The listing builds one solid part. Answer for the finished solid, in the listing's coordinates (mm). A direction names the side the tool comes from. Coordinates: 2 decimals unless noted, no trailing zeros. Order: outer loops, then holes, each group sorted by start corner. A loop starts at its lowest first (then second) coordinate and runs counter-clockwise, first axis right, second up.
```python
from build123d import *

# Parameters (mm, degrees)
FLANGE_HOLES_D    = 2.8702
DOWEL_HOLES_D     = 4.7625
DOWEL_HOLES_DEPTH = 6.35
DOWEL_HOLES_TIP   = 1.430799349
FILLET1_R         = 8.89
CHAMFER1_SIZE     = 2.141545552
CHAMFER1_SIZE_2   = 2.54


with BuildPart() as part:
    # Sketch2 → Main Structure (revolve)
    with BuildSketch(Plane.XY, mode=Mode.PRIVATE) as main_structure_sk:
        Polygon((0, 20.583496156), (0, 56.35625), (9.525, 56.35625), (9.525, 16.256), (66.806461084, 16.256), (139.7, 31.75), (139.7, 29.592458901), (60.325, 12.720781818), (60.325, 14.351), (10.795, 14.351), align=None)
    revolve(main_structure_sk.sketch.rotate(Axis((0, 0, 0), (1, 0, 0)), 90), axis=Axis((0, 0, 0), (1, 0, 0)))

    # Flange Holes (through all)
    with Locations(Plane.ZY):
        with Locations((0, -51.6255), (-25.81275, -44.708994483), (-44.708994483, -25.81275), (-51.6255, 0), (-44.708994483, 25.81275), (-25.81275, 44.708994483), (0, 51.6255), (25.81275, 44.708994483), (44.708994483, 25.81275), (51.6255, 0), (44.708994483, -25.81275), (25.81275, -44.708994483)):
            Hole(FLANGE_HOLES_D / 2)

    # Dowel Holes
    with Locations(Plane.ZY):
        with Locations((49.866403745, -13.361662613), (-49.866403745, 13.361662613)):
            Hole(DOWEL_HOLES_D / 2, depth=DOWEL_HOLES_DEPTH)
            with Locations((0, 0, -(DOWEL_HOLES_DEPTH + DOWEL_HOLES_TIP / 2))):  # 118° drill point
                Cone(0, DOWEL_HOLES_D / 2, DOWEL_HOLES_TIP, mode=Mode.SUBTRACT)

    # Fillet1
    fillet1_edges = [part.edges().sort_by_distance(p)[0] for p in [
        (66.806461084, 0, -16.256),
        (9.525, 0, -16.256),
    ]]
    fillet(fillet1_edges, radius=FILLET1_R)

    # Sketch13 → Cut-Revolve1 (revolve, cut)
    with BuildSketch(Plane(origin=(0, 0, 0), x_dir=(1, 0, 0), z_dir=(0, 1, 0)), mode=Mode.PRIVATE) as cut_revolve1_sk:
        Polygon((0, 38.1), (3.33331808, 0), (0, 0), align=None)
    revolve(cut_revolve1_sk.sketch.rotate(Axis((3.33331808, 0, 0), (-1, 0, 0)), 180), axis=Axis((3.33331808, 0, 0), (-1, 0, 0)), mode=Mode.SUBTRACT)

    # Chamfer1
    # the kernel refuses this chamfer: 3.297690964, 2.54, 2.141545552 mm, written as the material it takes off along each edge
    with BuildSketch(Plane(origin=(139.7, 0, 0), x_dir=(0, 0, 1), z_dir=(0, 1, 0))) as chamfer1_piece_1:
        Polygon((31.75 - CHAMFER1_SIZE * 0.207911690799, -CHAMFER1_SIZE * 0.978147600645), (31.75 - CHAMFER1_SIZE_2, 0), (31.75, 0), align=None)
    revolve(axis=Axis((139.7, 0, 0), (1, 0, 0)), mode=Mode.SUBTRACT)


solid = part.part
```
(1) Find section B-B (x = 16.5). Write down the section's boundary in (y, z), and give its area (3 significant figures).
(2) Each of these flat-tipped pins is pushed along its axis until it touches: pin 1 Ø10 at (y, z) = (-4, 13.5) entering from -X; pin 2 Ø23 at (y, z) = (4, -5.5) entering from -X; pin 3 Ø2.5 at (y, z) = (25.81, 44.71) entering from +X; pin 4 Ø4.5 at (y, z) = (25.81, -44.71) entering from +X (3 decimals). Where does it stop, or does it pass through?
(3) Find section A-A (x = 85). Write down the section's boundary in (y, z).
(4) The mould has two halves that part along Y. Classify faces 1 (the face through (9.525, 12, 24)), 2 (the face through (4.829, 34.292, -44.722)), 3 (the face through (60.325, 13, 1)): released by +Y, released by -Y, zero draft, split by the parting line, or undercut.
(5) Consider line 1 (X direction, y = -33, z = 18.5) (3 decimals); line 2 (Y direction, x = 68.5, z = 10); line 3 (Z direction, x = 43.5, y = 6). Determine where each line is inside the solid, lowest interval first.
(6) For faces 4 (the face through (99.3, 12.78, -16.67)), 5 (the face through (3.22, -11.35, 48.59)), 6 (the face through (95.387, 19.811, 10.304)), determine the directions among +Z, -Z, +X, -X, +Y, -Y from which every point of the face is accessible in a straight line to the end or side of a thin tool.
Findings below:
1. outline: circle Ø32.93 at (0, 0); hole circle Ø28.7 at (0, 0)
1. area: 205 mm2
2. pin 1: stops at x = 2.6
2. pin 2: stops at x = 3.95
2. pin 3: passes through
2. pin 4: stops at x = 9.525
3. outline: circle Ø40.25 at (0, 0); hole circle Ø35.93 at (0, 0)
4. face 1: zero draft
4. face 2: split by the parting line
4. face 3: undercut
5. line 1: x = 0.023 to 9.525
5. line 2: y = -13.27 to -10.44, 10.44 to 13.27
5. line 3: z = -15.11 to -13.04, 13.04 to 15.11
6. face 4: +X
6. face 5: -X
6. face 6: none
